The listing builds one solid part. Answer for the finished solid, in the listing's coordinates (mm). A direction names the side the tool comes from. Give positions to 0.01 mm unless a question says otherwise; leave off trailing zeros. Loops run counter-clockwise (first coordinate to the right, second up) from the corner with the lowest first, then second, coordinate; pieces in that order, holes last. Notation, with made-up numbers: M 35,82 L 73,82 A20 cw 73,98 Z; hole C 41.25,79 d11. An arc over 180 degrees is marked long. Use one line per item in the form item = value. Start each with the question number.
1. Straight lines are drawn through the part: line 1 (Z direction, x = 5.6, y = 2.3); line 2 (Z direction, x = 5.6, y = 1.3); line 3 (Z direction, x = 2.75, y = -0.25). For each, find the intervals that lie inside material, in ascending order. Write a range as from..to.
2. The part is cut by section C-C (y = 9.25). Write down the section's boundary in (x, z).
3. The part is cut by section A-A (y = -0.5). Write down the section's boundary in (x, z), and give its area (3 significant figures).
4. The part is cut by section B-B (z = 15). Write down the section's boundary in (x, y).
5. For faces 4 (the face through (6, 1.6, 9)), 5 (the face through (1.4, -6, 29)), 6 (the face through (-6, 7.369, 9)), 7 (the face through (3, 5, 9)), 8 (the face through (0.301, -4.289, 20.835)), determine the directions among +Z, -Z, +X, -X, +Y, -Y from which every point of the face is accessible in a straight line to the end or side of a thin tool.
6. The part is cut by section D-D (y = -5). Write down the section's boundary in (x, z), and give its area (3 significant figures).
7. Each of these flat-tipped pins is pushed along its axis until it touches: pin 1 Ø6 at (y, z) = (-1, 0.5) entering from -X; pin 2 Ø6.5 at (x, z) = (5.5, 0.5) entering from -Y; pin 3 Ø0.7 at (x, y) = (4, 5) entering from -Z. Where does it stop, or does it pass through?
8. The mould has two halves that part along Z. Classify faces 1 (the face through (5, -7.1, 24)), 2 (the face through (7, 2, 21.7)), 3 (the face through (-6.402, 9, 9)): released by +Z, released by -Z, zero draft, split by the parting line, or undercut.
from build123d import *

# Parameters (mm, degrees)
EXTRUSION1_DEPTH                                  = 18.1
COQUE1_START                                      = 1.2
COQUE1_DEPTH                                      = 15.7
EXTRUSION2_DEPTH                                  = 3.1
ESQUISSE3_W                                       = 6.2
ESQUISSE3_H                                       = 18.1
EXTRUSION3_DEPTH                                  = 1.9
CHAMBRAGE_POUR_VIS_T_TE_HEXAGONALE_M2_D           = 2.3
CHAMBRAGE_POUR_VIS_T_TE_HEXAGONALE_M2_CBORE_D     = 4.5
CHAMBRAGE_POUR_VIS_T_TE_HEXAGONALE_M2_CBORE_DEPTH = 1.8
ENL_V_MAT_EXTRU_1_DEPTH                           = 1.6
EXTRUSION4_DEPTH                                  = 1.6
R_P_TITION_LIN_AIRE1_COUNT                        = 2
R_P_TITION_LIN_AIRE1_PITCH                        = 9
EXTRUSION5_DEPTH                                  = 8
EXTRUSION5_DIRECTION_2_REACH                      = 27.934
ENL_V_MAT_EXTRU_2_DEPTH                           = 23.973967556
EXTRUSION6_DEPTH                                  = 11.8
EXTRUSION7_DEPTH                                  = 9.6
CHANFREIN1_SIZE                                   = 1
ESQUISSE12_W                                      = 3.65
ESQUISSE12_H                                      = 8.7
ENL_V_MAT_EXTRU_3_DEPTH                           = 32.201293006
EXTRUSION8_DEPTH                                  = 3.2
ESQUISSE14_W                                      = 6.4
ESQUISSE14_H                                      = 3.1
ENL_V_MAT_EXTRU_4_DEPTH                           = 1.6
CONG_1_R                                          = 1
CONG_2_R                                          = 1


# Read off the part's stored shape, not the designer's step: Coque1
with BuildPart() as part:
    # Esquisse1 → Extrusion1 (new body)
    with BuildSketch(Plane.XY):
        with BuildLine():
            Line((0.5, 0), (9.2, 0))
            Line((9.2, 0), (9.2, 3.1))
            Line((9.2, 3.1), (3, 3.1))
            Line((3, 3.1), (3, 6.1))
            Line((3, 6.1), (0.698275932, 10.81853434))
            Line((0.698275932, 10.81853434), (-5.901724068, 10.81853434))
            ThreePointArc((-5.901724068, 10.81853434), (-6.255277459, 10.67208773), (-6.401724068, 10.31853434))
            Line((-6.401724068, 10.31853434), (-6.401724068, 7.36853434))
            Line((-6.401724068, 7.36853434), (-5.101724068, 7.36853434))
            ThreePointArc((-5.101724068, 7.36853434), (-4.748170678, 7.514980949), (-4.601724068, 7.86853434))
            Line((-4.601724068, 7.86853434), (-4.601724068, 8.56853434))
            Line((-4.601724068, 8.56853434), (-3.201724068, 8.56853434))
            Line((-3.201724068, 8.56853434), (-3.201724068, 7.86853434))
            ThreePointArc((-3.201724068, 7.86853434), (-3.055277459, 7.514980949), (-2.701724068, 7.36853434))
            Line((-2.701724068, 7.36853434), (-1.301724068, 7.36853434))
            Line((-1.301724068, 7.36853434), (0, 4.7))
            Line((0, 4.7), (0, 0.5))
            ThreePointArc((0, 0.5), (0.146446609, 0.146446609), (0.5, 0))
        make_face()
    extrude(amount=EXTRUSION1_DEPTH)

    # Coque1 outline → Coque1 (cut)
    with BuildSketch(Plane.XY.offset(COQUE1_START)):
        with BuildLine():
            Line((-5.201724068, 8.56853434), (-3.201724068, 8.56853434))
            Line((-3.201724068, 8.56853434), (-3.201724068, 7.86853434))
            ThreePointArc((-3.201724068, 7.86853434), (-3.055277459, 7.514980949), (-2.701724068, 7.36853434))
            Line((-2.701724068, 7.36853434), (-1.301724068, 7.36853434))
            Line((-1.301724068, 7.36853434), (0, 4.7))
            Line((0, 4.7), (0, 0.5))
            ThreePointArc((0, 0.5), (0.146446609, 0.146446609), (0.5, 0))
            Line((0.5, 0), (8, 0))
            Line((8, 0), (8, 1.9))
            Line((8, 1.9), (1.8, 1.9))
            Line((1.8, 1.9), (1.8, 5.822921265))
            Line((1.8, 5.822921265), (-0.051518573, 9.61853434))
            Line((-0.051518573, 9.61853434), (-5.201724068, 9.61853434))
            Line((-5.201724068, 9.61853434), (-5.201724068, 8.56853434))
        make_face()
    extrude(amount=COQUE1_DEPTH, mode=Mode.SUBTRACT)

    # Esquisse2 → Extrusion2 (add)
    with BuildSketch(Plane(origin=(0, 3.1, 0), x_dir=(-1, 0, 0), z_dir=(0, 1, 0))):
        with BuildLine():
            Line((-9.2, 0), (-2, 0))
            ThreePointArc((-2, 0), (-5.6, -3.6), (-9.2, 0))
        make_face()
        with BuildLine():
            Line((-9.2, 18.1), (-2, 18.1))
            ThreePointArc((-2, 18.1), (-5.6, 21.7), (-9.2, 18.1))
        make_face()
    extrude(amount=-EXTRUSION2_DEPTH)

    # Esquisse3 → Extrusion3 (add)
    with BuildSketch(Plane.XZ):
        with Locations((4.9, 9.05)):
            Rectangle(ESQUISSE3_W, ESQUISSE3_H)
    extrude(amount=-EXTRUSION3_DEPTH)

    # Chambrage pour vis à tête hexagonale M2.51 (through all)
    with Locations(Plane.XZ):
        with Locations((5.6, 1.3), (5.6, 16.8)):
            CounterBoreHole(CHAMBRAGE_POUR_VIS_T_TE_HEXAGONALE_M2_D / 2, CHAMBRAGE_POUR_VIS_T_TE_HEXAGONALE_M2_CBORE_D / 2, CHAMBRAGE_POUR_VIS_T_TE_HEXAGONALE_M2_CBORE_DEPTH)

    # Esquisse6 → Enlèv. mat.-Extru.1 (cut)
    with BuildSketch(Plane.XZ):
        with BuildLine():
            Line((3.75, 4.9), (7.45, 4.9))
            ThreePointArc((7.45, 4.9), (7.803553391, 5.046446609), (7.95, 5.4))
            Line((7.95, 5.4), (7.95, 12.7))
            ThreePointArc((7.95, 12.7), (7.803553391, 13.053553391), (7.45, 13.2))
            Line((7.45, 13.2), (3.75, 13.2))
            ThreePointArc((3.75, 13.2), (3.396446609, 13.053553391), (3.25, 12.7))
            Line((3.25, 12.7), (3.25, 5.4))
            ThreePointArc((3.25, 5.4), (3.396446609, 5.046446609), (3.75, 4.9))
        make_face()
    extrude(amount=-ENL_V_MAT_EXTRU_1_DEPTH, mode=Mode.SUBTRACT)

    # Esquisse7 → Extrusion4 (add)
    with BuildSketch(Plane.XY.offset(14.35)):
        Polygon((3, 6.1), (5.3, 3.1), (3, 3.1), align=None)
    extrusion4 = extrude(amount=-EXTRUSION4_DEPTH)

    # Répétition linéaire1: Extrusion4 ×2
    with Locations(*[(0, 0, -i * R_P_TITION_LIN_AIRE1_PITCH) for i in range(1, R_P_TITION_LIN_AIRE1_COUNT)]):
        add(extrusion4)

    # Esquisse8 → Extrusion5 (add)
    with BuildSketch(Plane.XZ):
        Polygon((10.8, 4.55), (1.8, 4.55), (1.8, 5.95), (7.95, 5.95), (7.95, 12.15), (1.8, 12.15), (1.8, 13.55), (10.8, 13.55), (10.8, 12.15), (9.2, 12.15), (9.2, 5.95), (10.8, 5.95), align=None)
    extrude(amount=EXTRUSION5_DEPTH)

    # Extrusion5 direction 2: up to this face of the body (flat: up to its plane)
    extrusion5_direction_2_end = Plane(part.part.faces().sort_by_distance((6.086516905, 3.1, 9.05))[0])
    # Esquisse8 → Extrusion5 direction 2 (add, up to the picked face)
    with BuildSketch(Plane.XZ, mode=Mode.PRIVATE) as extrusion5_direction_2_sk1:
        Polygon((10.8, 4.55), (1.8, 4.55), (1.8, 5.95), (7.95, 5.95), (7.95, 12.15), (1.8, 12.15), (1.8, 13.55), (10.8, 13.55), (10.8, 12.15), (9.2, 12.15), (9.2, 5.95), (10.8, 5.95), align=None)
    extrusion5_direction_2_tool1 = split(extrude(extrusion5_direction_2_sk1.sketch, amount=-EXTRUSION5_DIRECTION_2_REACH, mode=Mode.PRIVATE), bisect_by=extrusion5_direction_2_end, keep=Keep.BOTH, mode=Mode.PRIVATE)
    add(extrusion5_direction_2_tool1.solids().sort_by(Axis((6.3, 0, 4.677279), (0, 1, 0)))[0])

    # Esquisse9 → Enlèv. mat.-Extru.2 (cut, through all)
    with BuildSketch(Plane(origin=(0, 0, 4.55), x_dir=(-1, 0, 0), z_dir=(0, 0, -1))):
        Polygon((-6.9, -8), (-1.8, -8), (-1.8, -1.6), align=None)
        Polygon((-10.8, 3.1), (-10.8, 1.5), (-9.3, 3.1), align=None)
    extrude(amount=-ENL_V_MAT_EXTRU_2_DEPTH, mode=Mode.SUBTRACT)

    # Esquisse10 → Extrusion6 (add)
    with BuildSketch(Plane(origin=(0, 3.1, 0), x_dir=(-1, 0, 0), z_dir=(0, 1, 0))):
        with BuildLine():
            Line((-9.2, 17.467725461), (-9.2, 27.2))
            Line((-9.2, 27.2), (-7.8, 27.2))
            Line((-7.8, 27.2), (-7.8, 21.7))
            Line((-7.8, 21.7), (-5.6, 21.7))
            ThreePointArc((-5.6, 21.7), (-3.054415588, 20.645584412), (-2, 18.1))
            Line((-2, 18.1), (-1.4, 18.1))
            Line((-1.4, 18.1), (-1.4, 27.2))
            Line((-1.4, 27.2), (0, 27.2))
            Line((0, 27.2), (0, 16.9))
            Line((0, 16.9), (-1.097371231, 16.9))
            Line((-1.097371231, 16.9), (-5.6, 19.545108536))
            Line((-5.6, 19.545108536), (-9.2, 17.467725461))
        make_face()
    extrude(amount=-EXTRUSION6_DEPTH)

    # Esquisse11 → Extrusion7 (add)
    with BuildSketch(Plane(origin=(0, 0.9, 0), x_dir=(-1, 0, 0), z_dir=(0, 1, 0))):
        with BuildLine():
            Line((-1.4, 22.7), (-1.4, 18.1))
            Line((-1.4, 18.1), (-2, 18.1))
            ThreePointArc((-2, 18.1), (-3.054415588, 20.645584412), (-5.6, 21.7))
            Line((-5.6, 21.7), (-7.8, 21.7))
            Line((-7.8, 21.7), (-7.8, 22.7))
            Line((-7.8, 22.7), (-1.4, 22.7))
        make_face()
    extrude(amount=-EXTRUSION7_DEPTH)

    # Chanfrein1
    chanfrein1_edges = [part.edges().sort_by_distance(p)[0] for p in [
        (4.6, 0.9, 22.7),
    ]]
    chamfer(chanfrein1_edges, length=CHANFREIN1_SIZE - 0.0001)  # a hair under: the kernel refuses the full size

    # Esquisse12 → Enlèv. mat.-Extru.3 (cut, through all)
    with BuildSketch(Plane.ZY):
        with Locations((18.725, -4.35)):
            Rectangle(ESQUISSE12_W, ESQUISSE12_H)
        Polygon((27.2, 3.1), (24.7, 3.1), (27.2, 0.6), align=None)
    extrude(amount=-ENL_V_MAT_EXTRU_3_DEPTH, mode=Mode.SUBTRACT)

    # Esquisse13 → Extrusion8 (add)
    with BuildSketch(Plane.XZ.offset(8.7)):
        with BuildLine():
            Line((9.2, 20.55), (0, 20.55))
            Line((0, 20.55), (0, 32.95))
            ThreePointArc((0, 32.95), (0.292893219, 33.657106781), (1, 33.95))
            Line((1, 33.95), (9.2, 33.95))
            Line((9.2, 33.95), (10.5, 33.95))
            ThreePointArc((10.5, 33.95), (11.207106781, 33.657106781), (11.5, 32.95))
            Line((11.5, 32.95), (11.5, 26.95))
            ThreePointArc((11.5, 26.95), (11.207106781, 26.242893219), (10.5, 25.95))
            Line((10.5, 25.95), (9.2, 25.95))
            Line((9.2, 25.95), (9.2, 20.55))
        make_face()
    extrude(amount=-EXTRUSION8_DEPTH)

    # Esquisse14 → Enlèv. mat.-Extru.4 (cut)
    with BuildSketch(Plane(origin=(0, -5.5, 0), x_dir=(-1, 0, 0), z_dir=(0, 1, 0))):
        with BuildLine():
            Line((-10.1, 27.2), (-1.4, 27.2))
            Line((-1.4, 27.2), (-1.4, 31.55))
            ThreePointArc((-1.4, 31.55), (-1.692893219, 32.257106781), (-2.4, 32.55))
            Line((-2.4, 32.55), (-10.1, 32.55))
            Line((-10.1, 32.55), (-10.1, 27.2))
        make_face()
        with Locations((-4.6, 24.25)):
            Rectangle(ESQUISSE14_W, ESQUISSE14_H)
    extrude(amount=-ENL_V_MAT_EXTRU_4_DEPTH, mode=Mode.SUBTRACT)

    # Congé1
    cong_1_edges = [part.edges().sort_by_distance(p)[0] for p in [
        (9.2, -4.35, 20.55),
        (0, -4.35, 20.55),
    ]]
    fillet(cong_1_edges, radius=CONG_1_R)

    # Congé2
    cong_2_edges = [part.edges().sort_by_distance(p)[0] for p in [
        (0, 2.35, 16.9),
    ]]
    fillet(cong_2_edges, radius=CONG_2_R)


solid = part.part
Derived:
q1.line_1 = -3.6..0.15, 2.45..15.65, 17.95..21.7
q1.line_2 = -3.6..-0.95, 3.55..5.95, 12.15..14.55, 19.05..21.7
q1.line_3 = 4.55..5.95, 12.15..13.55, 20.55..22.7
q2.outline = M -6.4,0 L 1.46,0 L 1.46,18.1 L -6.4,18.1 Z; hole M -5.2,1.2 L 0.13,1.2 L 0.13,16.9 L -5.2,16.9 Z
q3.outline = M 0,21.55 A1 ccw 1,20.55 L 8.2,20.55 A1 ccw 9.2,21.55 L 9.2,27.2 L 7.8,27.2 L 7.8,22.7 L 1.4,22.7 L 1.4,27.2 L 0,27.2 Z; M 1.8,4.55 L 10.8,4.55 L 10.8,5.95 L 9.2,5.95 L 9.2,12.15 L 10.8,12.15 L 10.8,13.55 L 1.8,13.55 L 1.8,12.15 L 7.95,12.15 L 7.95,5.95 L 1.8,5.95 Z
q3.area = 64.9 mm2
q4.outline = M -6.4,7.37 L -5.1,7.37 A0.5 ccw -4.6,7.87 L -4.6,8.57 L -5.2,8.57 L -5.2,9.62 L -0.05,9.62 L 1.8,5.82 L 1.8,0 L 4.25,0 L 4.25,1.8 L 6.95,1.8 L 6.95,0 L 9.2,0 L 9.2,3.1 L 3,3.1 L 3,6.1 L 0.7,10.82 L -5.9,10.82 A0.5 ccw -6.4,10.32 Z
q5.face_4 = -Y
q5.face_5 = +Y
q5.face_6 = +Z, -Z, -X, -Y
q5.face_7 = +X, +Y
q5.face_8 = -Z, -X, -Y
q6.outline = M 0,21.55 A1 ccw 1,20.55 L 8.2,20.55 A1 ccw 9.2,21.55 L 9.2,27.2 L 7.8,27.2 L 7.8,22.7 L 1.4,22.7 L 1.4,27.2 L 0,27.2 Z; M 4.51,4.55 L 10.8,4.55 L 10.8,5.95 L 9.2,5.95 L 9.2,12.15 L 10.8,12.15 L 10.8,13.55 L 4.51,13.55 L 4.51,12.15 L 7.95,12.15 L 7.95,5.95 L 4.51,5.95 Z
q6.area = 57.3 mm2
q7.pin_1 = 0
q7.pin_2 = 0
q7.pin_3 = 3.75
q8.face_1 = undercut
q8.face_2 = released by +Z
q8.face_3 = zero draft
